Here's the drawing with two shaded views (mm, measured from the low corner). I have some questions. Round coordinates to 2 decimals unless told otherwise and drop trailing zeros. Order: outer loops, then holes, each group sorted by start corner. A loop starts at its lowest first (then second) coordinate and runs counter-clockwise, first axis right, second up. Notation, with made-up numbers: (81, -5.75) -> (86, -5.75) arc R31 cw to (86, 19.25) -> close; hole circle Ø4 at (8.25, -23). An arc over 180 degrees is marked (long way). Answer in a Markdown table with one row per item.
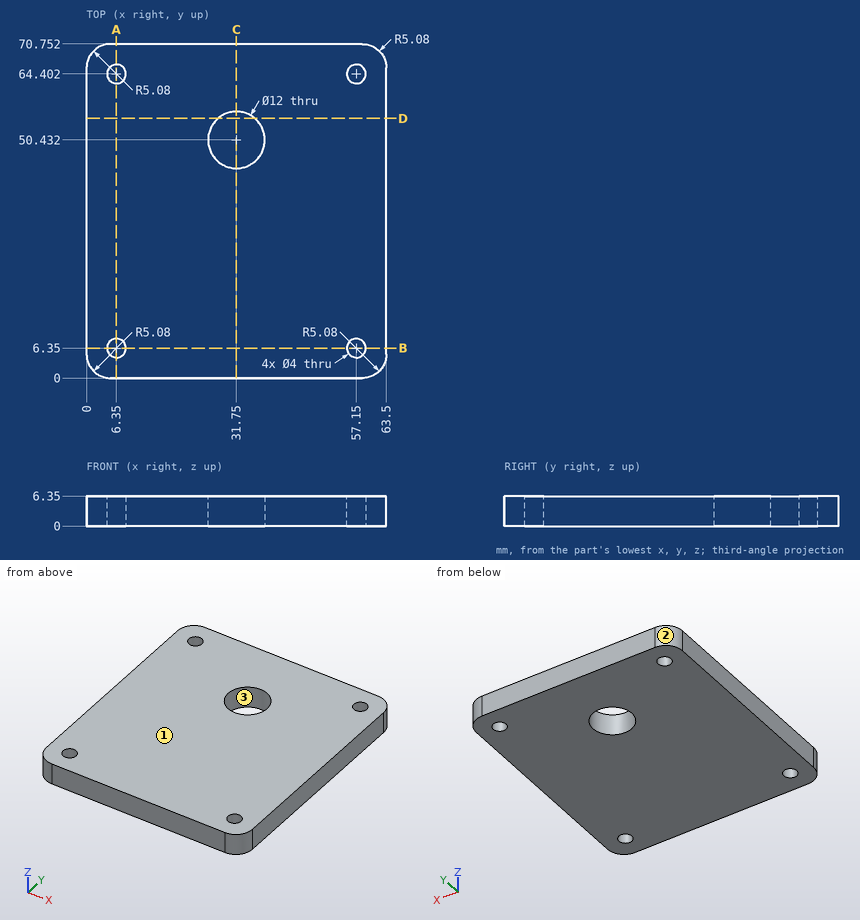
1. Suppose I cut it at A-A on x = 6.35. Write out the boundary of the cut face in (y, z).
Numbers:
| item | result |
|---|---|
| outline | (0, 0) -> (4.35, 0) -> (4.35, 6.35) -> (0, 6.35) -> close; (8.35, 0) -> (62.4, 0) -> (62.4, 6.35) -> (8.35, 6.35) -> close; (66.4, 0) -> (70.75, 0) -> (70.75, 6.35) -> (66.4, 6.35) -> close |
2. We'd pull the mould along X, two halves only. Please class the marked faces 1, 2 and 3: released by +X, released by -X, zero draft, split by the parting line, or undercut.
Numbers:
| item | result |
|---|---|
| face 1 | zero draft |
| face 2 | released by -X |
| face 3 | undercut |
3. Please list where these lines run through material, in increasing order: line 1 along Y through (x, z) = (57.15, 1.5); line 2 along Y through (x, z) = (8, 4); line 3 along Y through (x, z) = (32.5, 1.75) (1 decimal).
Numbers:
| item | result |
|---|---|
| line 1 | y = 0 to 4.35, 8.35 to 62.4, 66.4 to 70.75 |
| line 2 | y = 0 to 5.22, 7.48 to 63.27, 65.53 to 70.75 |
| line 3 | y = 0 to 44.5, 56.4 to 70.8 |
4. Suppose I cut it at D-D on y = 55. Write out the boundary of the cut face in (x, z), then the cut area to 3 significant figures.
Numbers:
| item | result |
|---|---|
| outline | (0, 0) -> (27.86, 0) -> (27.86, 6.35) -> (0, 6.35) -> close; (35.64, 0) -> (63.5, 0) -> (63.5, 6.35) -> (35.64, 6.35) -> close |
| area | 354 mm2 |
5. Suppose I cut it at C-C on x = 31.75. Write out the boundary of the cut face in (y, z), then the cut area to 3 significant figures.
Numbers:
| item | result |
|---|---|
| outline | (0, 0) -> (44.43, 0) -> (44.43, 6.35) -> (0, 6.35) -> close; (56.43, 0) -> (70.75, 0) -> (70.75, 6.35) -> (56.43, 6.35) -> close |
| area | 373 mm2 |
6. Suppose I cut it at B-B on y = 6.35. Write out the boundary of the cut face in (x, z).
Numbers:
| item | result |
|---|---|
| outline | (0, 0) -> (4.35, 0) -> (4.35, 6.35) -> (0, 6.35) -> close; (8.35, 0) -> (55.15, 0) -> (55.15, 6.35) -> (8.35, 6.35) -> close; (59.15, 0) -> (63.5, 0) -> (63.5, 6.35) -> (59.15, 6.35) -> close |
7. For pin 1 Ø3 at (x, y) = (6.35, 6.35) entering from +Z, with a flat end and sliding along its axis, tell me the tip position at first contact or that it passes through.
Numbers:
| item | result |
|---|---|
| pin 1 | passes through |
